Autodesk Inventor part; units mm, degrees
ref_plane "Work Plane1" through (-17.5, 9.4, 0) normal (1, 0, 0) x (0, 0, -1)
ref_plane "YZ Plane" through (0, 0, 0) normal (1, 0, 0) x (0, 1, 0)
ref_plane "XZ Plane" through (0, 0, 0) normal (0, 1, 0) x (-1, 0, 0)
sketch "Sketch1" plane through (0, 0, 0) normal (0, 0, 1) x (1, 0, 0)
  line L0 (-7.5, -9) -> (7.5, -9)
  line L1 (7.5, -9) -> (7.5, 9)
  line L2 (7.5, 9) -> (-7.5, 9)
  line L3 (-9.5, -11) -> (-9.5, -12.75)
  line L4 (-12.5, -15.75) -> (-17.5, -15.75)
  arc A0 (-7.5, -9) -> (-9.5, -11) centre (-7.5, -11) ccw
  line L5 (-12.5, -15.75) -> (-9.5, -12.75)
  line L6 (-17.5, -15.75) -> (-17.5, -6.1)
  line L7 (-17.5, -6.1) -> (-13.3, -6.1)
  line L8 (-13.3, -6.1) -> (-13.3, 0)
  line L9 (2.7531, 0) -> (-2.7531, 0) construction
  line L10 (-9.5, 11) -> (-9.5, 12.75)
  line L11 (-12.5, 15.75) -> (-17.5, 15.75)
  arc A1 (-9.5, 11) -> (-7.5, 9) centre (-7.5, 11) ccw
  line L12 (-12.5, 15.75) -> (-9.5, 12.75)
  line L13 (-17.5, 15.75) -> (-17.5, 6.1)
  line L14 (-17.5, 6.1) -> (-13.3, 6.1)
  line L15 (-13.3, 6.1) -> (-13.3, 0)
  circle A2 centre (-14, -11.75) radius 1.575
  circle A3 centre (-14, 11.75) radius 1.575
  line L16 (-17.5, 15.75) -> (-23.85, 15.75)
  line L17 (-23.85, 15.75) -> (-23.85, 9.4)
  line L18 (-23.85, 9.4) -> (-17.5, 9.4)
  line L19 (-9.5, 11.875) -> (-9.5, -11.875)
  point P0 (0, 0)
  point P1 (0, 0)
  point P2 (7.5, 0)
  point P3 (0, -9)
  point P4 (-9.5, -15.75)
  point P5 (0, 0)
  point P6 (-9.5, 15.75)
  dimension "d1" = 18
  dimension "d3" = 8
  dimension "d4" = 2
  dimension "d5" = 3
  dimension "d6" = 3
  dimension "d7" = 9.65
  dimension "d8" = 4.2
  dimension "d9" = 6.1
  dimension "d10" = 7.5
  dimension "d11" = 3.875
  dimension "d12" = 3.15
  dimension "d13" = 3.5
  dimension "d14" = 4
  dimension "d15" = 6.35
  dimension "d16" = 6.35
extrude "Extrusion1" add sketch "Sketch1" against normal blind 15 contours L3 L5 L4 L6 L7 L8 L15 L14 L13 L11 L12 L10 L19
extrude "Extrusion2" add sketch "Sketch1" against normal blind 13.291 contours A0 L19 A1 L2 L1 L0
chamfer "Chamfer1" distance 17 distance2 8.281 1 edges at (7.5, 0, -13.291) measured on face at (-2.5, 3, -13.291)
extrude "Extrusion3" add sketch "Sketch1" along normal blind 15.861 and the other way blind 15 contours L13 L18 L17 L16
ref_plane "Work Plane1" through (-17.5, 9.4, 0) normal (1, 0, 0) x (0, 0, -1)
sketch "Sketch2" plane through (-17.5, 9.4, 0) normal (1, 0, 0) x (0, 0, -1)
  line L0 (0, 6.35) -> (0, 0)
  line L1 (15, 0) -> (0, 0)
  line L2 (15, 6.35) -> (15, 0)
  line L3 (0, 6.35) -> (15, 6.35)
  line L4 (-15.861, 6.35) -> (0, 6.35)
  line L5 (-15.861, 0) -> (-15.861, 6.35)
  line L6 (0, 0) -> (-15.861, 0)
  line L7 (0, -3.3) -> (0, 0)
  line L8 (15, -3.3) -> (0, -3.3)
  line L9 (15, 0) -> (15, -3.3)
  line L10 (0, -15.5) -> (15, -15.5)
  line L11 (15, -15.5) -> (15, -25.15)
  line L12 (15, -25.15) -> (0, -25.15)
  line L13 (0, -25.15) -> (0, -15.5)
  line L14 (-15.861, 0) -> (-14.969, 0)
  line L15 (-14.969, 0) -> (-14.1416, 2.2732)
  line L16 (-14.1416, 2.2732) -> (-13.2496, 2.2732)
  line L17 (-13.2496, 2.2732) -> (-12.4223, 0)
  line L18 (-15.861, 0) -> (15, 0)
  line L19 (-9.8106, 2.2732) -> (-8.9833, 0)
  line L20 (-10.7026, 2.2732) -> (-9.8106, 2.2732)
  line L21 (-11.53, 0) -> (-10.7026, 2.2732)
  line L22 (-12.422, 0) -> (-11.53, 0)
  line L23 (-6.3716, 2.2732) -> (-5.5443, 0)
  line L24 (-7.2636, 2.2732) -> (-6.3716, 2.2732)
  line L25 (-8.091, 0) -> (-7.2636, 2.2732)
  line L26 (-8.983, 0) -> (-8.091, 0)
  line L27 (-2.9326, 2.2732) -> (-2.1053, 0)
  line L28 (-3.8246, 2.2732) -> (-2.9326, 2.2732)
  line L29 (-4.652, 0) -> (-3.8246, 2.2732)
  line L30 (-5.544, 0) -> (-4.652, 0)
  line L31 (0.5064, 2.2732) -> (1.3337, 0)
  line L32 (-0.3856, 2.2732) -> (0.5064, 2.2732)
  line L33 (-1.213, 0) -> (-0.3856, 2.2732)
  line L34 (-2.105, 0) -> (-1.213, 0)
  line L35 (3.9454, 2.2732) -> (4.7727, 0)
  line L36 (3.0534, 2.2732) -> (3.9454, 2.2732)
  line L37 (2.226, 0) -> (3.0534, 2.2732)
  line L38 (1.334, 0) -> (2.226, 0)
  line L39 (7.3844, 2.2732) -> (8.2117, 0)
  line L40 (6.4924, 2.2732) -> (7.3844, 2.2732)
  line L41 (5.665, 0) -> (6.4924, 2.2732)
  line L42 (4.773, 0) -> (5.665, 0)
  line L43 (10.8234, 2.2732) -> (11.6507, 0)
  line L44 (9.9314, 2.2732) -> (10.8234, 2.2732)
  line L45 (9.104, 0) -> (9.9314, 2.2732)
  line L46 (8.212, 0) -> (9.104, 0)
  line L47 (14.2624, 2.2732) -> (15.0897, 0)
  line L48 (13.3704, 2.2732) -> (14.2624, 2.2732)
  line L49 (12.543, 0) -> (13.3704, 2.2732)
  line L50 (11.651, 0) -> (12.543, 0)
  point P0 (0, -9.4)
  point P1 (15, 0.2465)
  point P2 (11.6507, 0)
  point P3 (8.2117, 0)
  point P4 (4.7727, 0)
  point P5 (1.3337, 0)
  point P6 (-2.1053, 0)
  point P7 (-5.5443, 0)
  point P8 (-8.9833, 0)
  point P9 (-12.4223, 0)
  dimension "d29" = 0.892
  dimension "d30" = 110
  dimension "d31" = 110
  dimension "d32" = 0.892
  dimension "d33" = 2.2732
  dimension "d36" = 3.439
extrude "Extrusion4" cut sketch "Sketch2" against normal up to surface (6.35 mm away) contours L32 L31 L1 L0 | L0 L6 L33 L32 | L2 L1 L49 L48 L47 | L15 L16 L17 L6 | L37 L36 L35 L1 | L6 L29 L28 L27 | L1 L45 L44 L43 | L21 L20 L19 L6 | L41 L40 L39 L1 | L6 L25 L24 L23
fillet "Fillet1" radius 0.2 35 edges at (-20.675, 11.6732, 14.1416) (-20.675, 11.6732, 13.2496) (-20.675, 9.4, 14.969) (-20.675, 9.4, 12.4223) (-20.675, 9.4, 11.53) (-20.675, 11.6732, 10.7026) (-20.675, 11.6732, 9.8106) (-20.675, 9.4, 8.9833) (-20.675, 9.4, 8.091) (-20.675, 11.6732, 7.2636) (-20.675, 11.6732, 6.3716) (-20.675, 9.4, 5.5443) (-20.675, 9.4, 4.652) (-20.675, 11.6732, 3.8246) (-20.675, 11.6732, 2.9326) (-20.675, 9.4, 2.1053) (-20.675, 9.4, 1.213) (-20.675, 11.6732, 0.3856) (-20.675, 11.6732, -0.5064) (-20.675, 9.4, -1.3337) (-20.675, 9.4, -2.226) (-20.675, 11.6732, -3.0534) (-20.675, 11.6732, -3.9454) (-20.675, 9.4, -4.7727) (-20.675, 9.4, -5.665) (-20.675, 11.6732, -6.4924) (-20.675, 11.6732, -7.3844) (-20.675, 9.4, -8.2117) (-20.675, 9.4, -9.104) (-20.675, 11.6732, -9.9314) (-20.675, 11.6732, -10.8234) (-20.675, 9.4, -11.6507) (-20.675, 9.4, -12.543) (-20.675, 11.6732, -13.3704) (-20.675, 11.6732, -14.2624)
properties part number "GA_1"
The model under review builds one solid part; all positions refer to its coordinate system, in mm. A direction names the side the tool comes from. Round coordinates to 2 decimals unless told otherwise and drop trailing zeros. Write each loop counter-clockwise with the first axis right and the second up, starting at its lowest first coordinate (ties: lowest second). Pieces come first, ordered by that corner, then holes. Notation, with made-up numbers: M 65.25,82.25 L 115.25,82.25 A16 ccw 115.25,89.25 Z; hole C -9,13 d8. An arc over 180 degrees is marked long. Use CSV: the item, a comma, the result in double quotes. Start each with the question number.
(1) The part is to be moulded in two halves that separate along Z. For faces 1 (the face through (-12, 4, -15)), 2 (the face through (-20.63, 10.55, 9.4)), 3 (the face through (-15, -6.1, -7)), say which applies: +Z half, -Z half, draft (parallel to the pull), parting line (faces both ways), or undercut.
(2) Clearance check with flat-ended pins moving along their axes: P1, Ø6, axis at x = -2, z = -4, coming from the +Y side; P2, Ø7.5, axis at y = 4, z = -10.5, coming from the +X side; P3, Ø10, axis at x = -6.5, y = 12.5, coming from the +Z side; P4, Ø1, axis at y = 8.5, z = 7.5, coming from the -X side. State where each tip first meets the part, or that it passes through.
(3) For line 1 along Y through (x, z) = (-14, -4.75) (3 decimals); line 2 along X through (y, z) = (11, -6); line 3 along Z through (x, y) = (-2.5, 7), list the stretches that pass through material, from the lowest coordinate up.
(4) We need section B-B, the plane x = -14. State the section outline as (y, z) points (3 decimals), then the cut area to 3 significant figures.
(5) Tool access review of faces 4 (the face through (-20.631, 10.551, -7.793)), 5 (the face through (7.5, 0, -2)), 6 (the face through (-20.631, 10.523, 0.804)), 7 (the face through (-2, 9, -5)): name each direction out of +Z, -Z, +X, -X, +Y, -Y from which nothing blocks a thin tool from reaching the whole face with its end or side.
(6) We need section D-D, the plane x = -1. State the section outline as (y, z) points, then the cut area to 3 significant figures.
(7) We need section A-A, the plane y = -11.75. State the section outline as (x, z) points (3 decimals).
Findings:
1,face 1,"-Z half"
1,face 2,"undercut"
1,face 3,"draft"
2,P1,"y = 9"
2,P2,"x = 3.93"
2,P3,"z = 0"
2,P4,"through"
3,line 1,"-15.75 to -13.325, -10.175 to -6.1, 6.1 to 10.175, 13.325 to 15.75"
3,line 2,"-23.85 to -15.38, -12.62 to -9.5"
3,line 3,"-9.88 to 0"
4,outline,"M -15.75,-15 L -13.325,-15 L -13.325,0 L -15.75,0 Z; M -10.175,-15 L -6.1,-15 L -6.1,0 L -10.175,0 Z; M 6.1,-15 L 10.175,-15 L 10.175,0 L 6.1,0 Z; M 13.325,-15 L 15.75,-15 L 15.75,0 L 13.325,0 Z"
4,area,"195 mm^2"
5,face 4,"-X, -Y"
5,face 5,"+Z, -Z, +X, +Y, -Y"
5,face 6,"+X, -X, -Y"
5,face 7,"+Z, -Z, +X, +Y"
6,outline,"M -9,-9.15 L 9,-9.15 L 9,0 L -9,0 Z"
6,area,"165 mm^2"
7,outline,"M -17.5,-15 L -15.575,-15 L -15.575,0 L -17.5,0 Z; M -12.425,-15 L -9.5,-15 L -9.5,0 L -12.425,0 Z"
